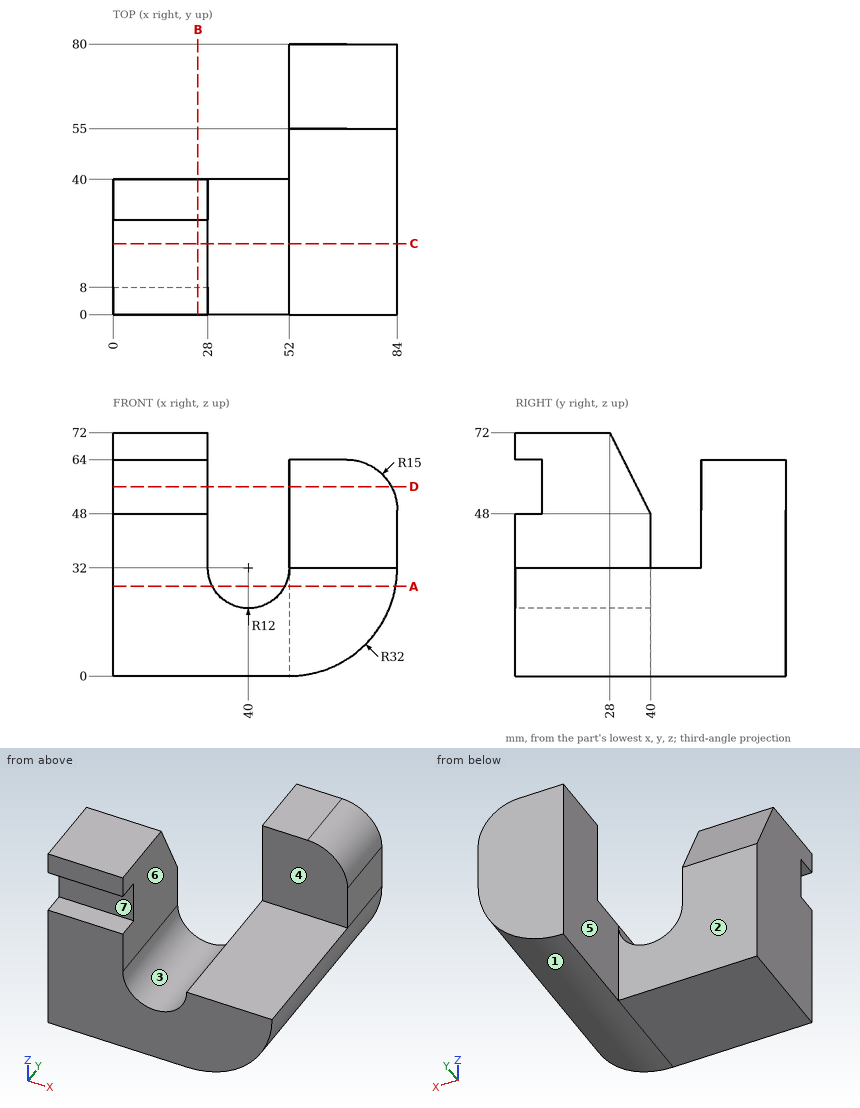
Design review of the part shown in the three views and the two pictorial views. Dimensions are in mm from the part's minimum x, y and z. A direction names the side the tool comes from. Round coordinates to 2 decimals unless told otherwise and drop trailing zeros. Order: outer loops, then holes, each group sorted by start corner. A loop starts at its lowest first (then second) coordinate and runs counter-clockwise, first axis right, second up. Notation, with made-up numbers: M 71,30 L 102,30 A28 cw 102,58 Z; hole C 86,35 d8. An arc over 180 degrees is marked long. Put each result on its own line as item: value.
Q1. Machinability: for the marked faces 4, 5, 6 and 7, which of the approach directions +Z, -Z, +X, -X, +Y, -Y give a long, thin tool a straight path to every point of the face, cutting with its end or side? Answer none if there is none.
Reported:
face 4: +Z, +X, -X, -Y
face 5: +Z, -Z, -X, +Y
face 6: +Z, +X, +Y, -Y
face 7: +X, -X, -Y
Q2. To check wall thickness, follow line 1 (Y direction, x = 51.5, z = 24.5); line 2 (X direction, y = 15, z = 51); line 3 (Y direction, x = 5, z = 55.5). State the ranges of each line that lie inside material, in increasing order.
Reported:
line 1: 0 to 40
line 2: 0 to 28
line 3: 8 to 36.25
Q3. Consider section A-A (z = 26.5). State the section outline as (x, y) points, and give its area (3 significant figures).
Reported:
outline: M 0,0 L 29.33,0 L 29.33,40 L 0,40 Z; M 50.67,0 L 83.52,0 L 83.52,80 L 52,80 L 52,40 L 50.67,40 Z
area: 3,750 mm²
Q4. Consider section D-D (z = 56). State the section outline as (x, y) points.
Reported:
outline: M 0,8 L 28,8 L 28,36 L 0,36 Z; M 52,55 L 82.27,55 L 82.27,80 L 52,80 Z
Q5. Insertion check: pin 1 Ø8 at (x, z) = (8, 55) entering from -Y; pin 2 Ø20 at (y, z) = (68.5, 47) entering from -X; pin 3 Ø5 at (y, z) = (22.5, 50) entering from +X. Each pin has a flat end and moves straight along its axis. Give the tip position at first contact, or say it passes through.
Reported:
pin 1: y = 8
pin 2: x = 52
pin 3: x = 28
Q6. Consider section B-B (x = 25). State the section outline as (y, z) points, and give its area (3 significant figures).
Reported:
outline: M 0,0 L 40,0 L 40,48 L 28,72 L 0,72 L 0,64 L 8,64 L 8,48 L 0,48 Z
area: 2,610 mm²
Q7. Consider section C-C (y = 21). State the section outline as (x, z) points.
Reported:
outline: M 0,0 L 52,0 A32 ccw 84,32 L 52,32 A12 cw 28,32 L 28,72 L 0,72 Z
Q8. Draft analysis for pull direction X (two halves, no side actions). For the marked faces 1, 2 and 3, state which applies: released by +X, released by -X, zero draft, split by the parting line, or undercut.
Reported:
face 1: released by +X
face 2: zero draft
face 3: undercut
